The model under review builds one solid part; all positions refer to its coordinate system, in mm. A direction names the side the tool comes from. Coordinates: 2 decimals unless noted, no trailing zeros. Order: outer loops, then holes, each group sorted by start corner. A loop starts at its lowest first (then second) coordinate and runs counter-clockwise, first axis right, second up.
```python
from build123d import *

# Parameters (mm, degrees)
PAD_DEPTH    = 8
POCKET_DEPTH = 4


with BuildPart() as part:
    # Sketch001 → Pad (new body)
    with BuildSketch(Plane.XY):
        with BuildLine():
            ThreePointArc((-34.447941, -1.81802), (-35.378998, -9.500456), (-28.560543, -13.160422))
            Line((-28.560543, -13.160422), (-23.837885, -11.246234))
            Line((-23.837885, -11.246234), (-19.304688, -9.234627))
            Line((-19.304688, -9.234627), (-14.743155, -7.818003))
            Line((-14.743155, -7.818003), (-10.096628, -6.826365))
            Line((-10.096628, -6.826365), (-6.951722, -6.373045))
            Line((-6.951722, -6.373045), (0, -6.373045))
            Line((6.951722, -6.373045), (0, -6.373045))
            Line((10.096628, -6.826365), (6.951722, -6.373045))
            Line((14.743155, -7.818003), (10.096628, -6.826365))
            Line((19.304688, -9.234627), (14.743155, -7.818003))
            Line((23.837885, -11.246234), (19.304688, -9.234627))
            Line((28.560543, -13.160422), (23.837885, -11.246234))
            ThreePointArc((28.560543, -13.160422), (35.378998, -9.500456), (34.447941, -1.81802))
            Line((34.447941, -1.81802), (27.67498, 4.071902))
            Line((27.67498, 4.071902), (20.478533, 8.265109))
            Line((20.478533, 8.265109), (13.112085, 10.843365))
            Line((13.112085, 10.843365), (5.802306, 12.344987))
            Line((5.802306, 12.344987), (0, 12.751387))
            Line((-5.802306, 12.344987), (0, 12.751387))
            Line((-13.112085, 10.843365), (-5.802306, 12.344987))
            Line((-20.478533, 8.265109), (-13.112085, 10.843365))
            Line((-27.67498, 4.071902), (-20.478533, 8.265109))
            Line((-34.447941, -1.81802), (-27.67498, 4.071902))
        make_face()
        with BuildLine():
            ThreePointArc((-19.507144, -4.931658), (-18.255876, -1.006404), (-22.181131, 0.244864))
            Line((-22.181131, 0.244864), (-30.233268, -3.914552))
            ThreePointArc((-30.233268, -3.914552), (-31.484536, -7.839806), (-27.559282, -9.091074))
            Line((-19.507144, -4.931658), (-27.559282, -9.091074))
        make_face(mode=Mode.SUBTRACT)
        with BuildLine():
            ThreePointArc((22.181131, 0.244864), (18.255876, -1.006404), (19.507144, -4.931658))
            Line((19.507144, -4.931658), (27.559282, -9.091074))
            ThreePointArc((27.559282, -9.091074), (31.484536, -7.839806), (30.233268, -3.914552))
            Line((22.181131, 0.244864), (30.233268, -3.914552))
        make_face(mode=Mode.SUBTRACT)
    extrude(amount=PAD_DEPTH)

    # Sketch003 → Pocket (cut)
    with BuildSketch(Plane.XY.offset(8)):
        Polygon((33.25967, -4.087808), (19.777759, 2.487759), (16.06826, -0.01433), (16.380383, -4.477895), (29.862294, -11.053462), (33.571793, -8.551373), align=None)
        Polygon((-33.25967, -4.087808), (-19.777759, 2.487759), (-16.06826, -0.01433), (-16.380383, -4.477895), (-29.862294, -11.053462), (-33.571793, -8.551373), align=None)
    extrude(amount=-POCKET_DEPTH, mode=Mode.SUBTRACT)


solid = part.part
```
(1) Draft analysis for pull direction X (two halves, no side actions). For faces 1 (the face through (16.847, 9.536, 3.944)), 2 (the face through (-17.949, 1.254, 6.028)), 3 (the face through (-1, 0, 8)), 4 (the face through (33.418, -6.351, 6.028)), state which applies: released by +X, released by -X, zero draft, split by the parting line, or undercut.
A:
face 1: released by +X
face 2: undercut
face 3: zero draft
face 4: undercut
(2) We need section A-A, the plane z = 1.75. Count the separate pieces of the cut face and the enclosed holes in it, and give its area (3 significant figures).
A:
separate pieces: 1
enclosed holes: 2
area: 1,050 mm2
(3) For pin 1 Ø2.5 at (x, z) = (-3, 3.5) entering from -Y; pin 2 Ø4 at (x, z) = (7, 4) entering from -Y; pin 3 Ø1.5 at (y, z) = (6, 4) entering from -X, all flat-tipped, find the tip position at first contact; note any pin that passes through.
A:
pin 1: stops at y = -6.37
pin 2: stops at y = -6.67
pin 3: stops at x = -25.65
(4) We need section C-C, the plane x = -1.5. Write out the cut boundary in (y, z).
A:
outline: (-6.37, 0) - (12.65, 0) - (12.65, 8) - (-6.37, 8) - close
(5) Machinability: for faces 5 (the face through (-24.127, 6.139, 3.944)), 6 (the face through (-23.03, -7.72, 6.03)), 7 (the face through (21.603, -10.255, 3.944)), 8 (the face through (23.477, -6.982, 1.972)), which of the approach directions +Z, -Z, +X, -X, +Y, -Y give a long, thin tool a straight path to every point of the face, cutting with its end or side? Answer none if there is none.
A:
face 5: +Z, -Z, -X, +Y
face 6: +Z
face 7: +Z, -Z, -Y
face 8: +Z, -Z
(6) We need section D-D, the plane y = 5.75. Write out the cut boundary in (x, z) (3 decimals).
A:
outline: (-24.795, 0) - (24.795, 0) - (24.795, 8) - (-24.795, 8) - close
(7) We need section B-B, the plane y = -1. Write out the cut boundary in (x, z), and give its area (3 significant figures).
A:
outline: (-33.51, 0) - (-24.59, 0) - (-24.59, 4) - (-26.93, 4) - (-26.93, 8) - (-33.51, 8) - close; (-18.26, 0) - (18.26, 0) - (18.26, 4) - (16.14, 4) - (16.14, 8) - (-16.14, 8) - (-16.14, 4) - (-18.26, 4) - close; (24.59, 0) - (33.51, 0) - (33.51, 8) - (26.93, 8) - (26.93, 4) - (24.59, 4) - close
area: 399 mm2
(8) Wall thickness on probe 1 along X at (y, z) = (-10.75, 4.5); probe 2 along X at (y, z) = (-4, 1.75); probe 3 along Y at (x, z) = (26, 0.5): over which ranges is each line inside the solid? List them lowest first.
A:
probe 1: x = -34.55 to -30.31, -29.24 to -22.72, 22.72 to 29.24, 30.31 to 34.55
probe 2: x = -35.74 to -30.39, -18.45 to 18.45, 30.39 to 35.74
probe 3: y = -12.12 to -8.29, -1.73 to 5.05
